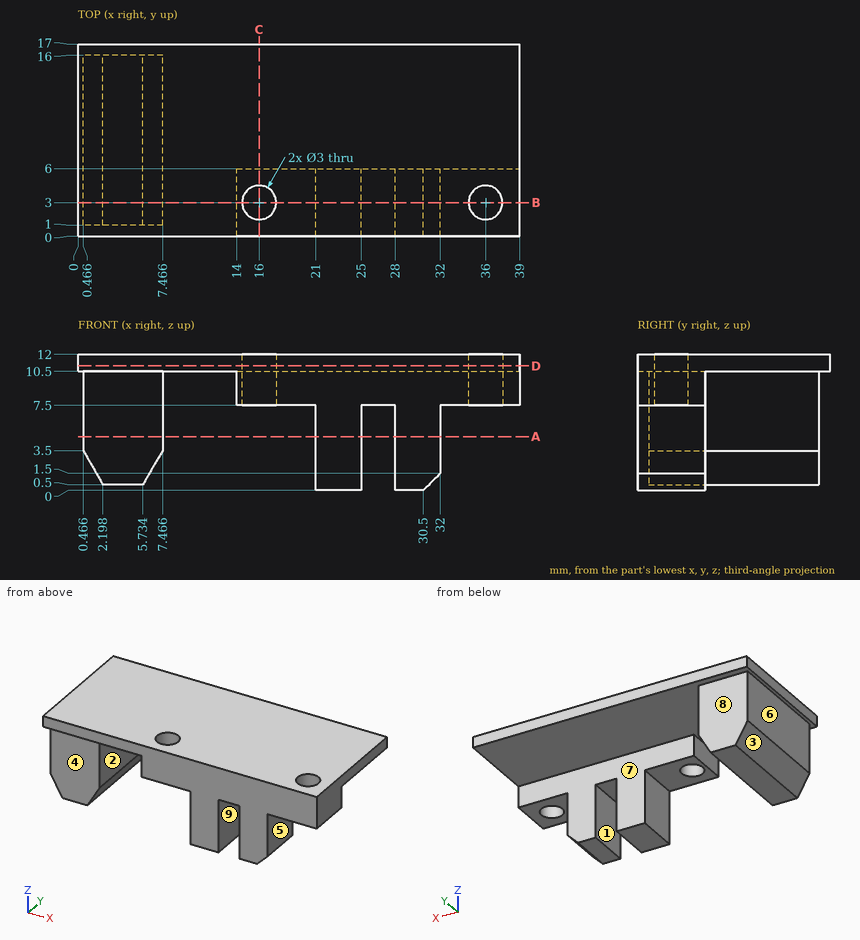
Design review of the part shown in the three views and the two pictorial views. Dimensions are in mm from the part's minimum x, y and z. A direction names the side the tool comes from. Coordinates: 2 decimals unless noted, no trailing zeros. Order: outer loops, then holes, each group sorted by start corner. A loop starts at its lowest first (then second) coordinate and runs counter-clockwise, first axis right, second up.
1) For the marked faces 5, 6, 7, 8 and 9, list the 3-axis set-ups (+Z, -Z, +X, -X, +Y, -Y) from which the entire face can be reached by the end or side of a thin tool; tool diameter is ignored.
2) Wall thickness on line 1 along X through (y, z) = (2, 6); line 2 along Y through (x, z) = (16, 10.8); line 3 along Z through (x, y) = (17, 10.5): over which ranges is each line inside the solid? List them lowest first.
3) Mouldability with a two-part tool opening along X and no side actions: class the marked faces 1, 2, 3 and 4 as +X half, -X half, draft (parallel to the pull), parting line (faces both ways), or undercut.
4) Take a section at C-C, the plane x = 16. Give the boundary of the cut face in (y, z).
5) Take a section at B-B, the plane y = 3. State how many separate pieces and enclosed holes the cut face has, and give its area (3 significant figures).
6) Take a section at D-D, the plane z = 11. Give the boundary of the cut face in (x, y), and give its area (3 significant figures).
7) Take a section at A-A, the plane z = 4.75. Give the boundary of the cut face in (x, y).
8) Clearance check with flat-ended pins moving along their axes: pin 1 (5.5 mm diameter, centred on y = 8.5, z = 5.5, fed in from -X); pin 2 (2 mm diameter, centred on x = 5, z = 5.5, fed in from +Y); pin 3 (4 mm diameter, centred on x = 20, y = 9, fed in from -Z); pin 4 (4 mm diameter, centred on x = 15, y = 3, fed in from +Z). State where each tip first meets the part, or that it passes through.
Returned:
1. face 5: -Z, +X, +Y, -Y
1. face 6: -Z, -X, +Y, -Y
1. face 7: -Z, +X, +Y
1. face 8: -Z, +X, -X, +Y
1. face 9: -Z, +Y, -Y
2. line 1: x = 0.47 to 7.47, 21 to 25, 28 to 32
2. line 2: y = 0 to 1.5, 4.5 to 17
2. line 3: z = 10.5 to 12
3. face 1: undercut
3. face 2: undercut
3. face 3: -X half
3. face 4: draft
4. outline: (0, 7.5) - (1.5, 7.5) - (1.5, 12) - (0, 12) - close; (4.5, 7.5) - (6, 7.5) - (6, 10.5) - (17, 10.5) - (17, 12) - (4.5, 12) - close
5. separate pieces: 3
5. enclosed holes: 0
5. area: 230 mm2
6. outline: (0, 0) - (39, 0) - (39, 17) - (0, 17) - close; hole circle Ø3 at (16, 3); hole circle Ø3 at (36, 3)
6. area: 649 mm2
7. outline: (0.47, 1) - (7.47, 1) - (7.47, 16) - (0.47, 16) - close; (21, 0) - (25, 0) - (25, 6) - (21, 6) - close; (28, 0) - (32, 0) - (32, 6) - (28, 6) - close
8. pin 1: stops at x = 0.47
8. pin 2: stops at y = 16
8. pin 3: stops at z = 10.5
8. pin 4: stops at z = 12
